Autodesk Inventor part; units mm, degrees
ref_plane "YZ Plane" through (0, 0, 0) normal (1, 0, 0) x (0, 1, 0)
ref_plane "XZ Plane" through (0, 0, 0) normal (0, 1, 0) x (-1, 0, 0)
ref_plane "XY Plane" through (0, 0, 0) normal (0, 0, 1) x (1, 0, 0)
sketch "Sketch1" plane through (0, 0, 0) normal (0, 0, 1) x (1, 0, 0)
  line L0 (0, 0) -> (20, 0)
  line L1 (20, 0) -> (20, 20)
  line L2 (20, 20) -> (0, 20)
  line L3 (0, 20) -> (0, 0)
  dimension "d0" = 20
  dimension "d1" = 20
extrude "Extrusion1" add sketch "Sketch1" along normal blind 20
sketch "Sketch2" plane through (0, 20, 0) normal (0, 1, 0) x (1, 0, 0)
  line L0 (20, 0) -> (0, 0)
  line L1 (20, 0) -> (20, -20)
  circle A0 centre (10, -5.8) radius 6.2
  dimension "d4" = 12.4
  dimension "d5" = 10
  dimension "d6" = 5.8
extrude "Extrusion2" cut sketch "Sketch2" against normal blind 20
sketch "Sketch5" plane through (0, 0, 0) normal (0, 0, -1) x (-1, 0, 0)
  line L0 (-12.1909, 0) -> (-12.1909, 20)
  line L1 (-20, 20) -> (-12.1909, 20)
  line L2 (-12.1909, 0) -> (-20, 0)
  line L3 (-16.2, 20) -> (-16.2, 0)
  point P0 (0, 0)
extrude "Extrusion3" cut sketch "Sketch5" against normal blind 5.8
sketch "Sketch6" plane through (0, 0, 0) normal (0, 0, -1) x (-1, 0, 0)
  line L0 (-7.8091, 20) -> (-7.8091, 0)
  line L1 (0, 0) -> (-7.8091, 0)
  line L2 (-7.8091, 20) -> (0, 20)
  line L3 (-3.8, 20) -> (-3.8, 0)
extrude "Extrusion4" cut sketch "Sketch6" against normal blind 5.8
properties part number "SupportBlocks"
Input: part model. Units: mm. Frame: model coordinates. A direction names the side the tool comes from. Coordinates: 2 decimals unless noted, no trailing zeros. Write each loop counter-clockwise with the first axis right and the second up, starting at its lowest first coordinate (ties: lowest second). Pieces come first, ordered by that corner, then holes. Notation, with made-up numbers: (3.25, 84.5) - (25.25, 84.5) arc R18 cw to (25.25, 94.5) - close; hole circle Ø5 at (63.25, 76). An arc over 180 degrees is marked (long way). Put each result on its own line as item: value. Start each with the question number.
1) Mould query, pull axis X, two halves, no side actions, for faces 3 (the face through (0, 10, 10)), 4 (the face through (3.8, 10, 3)), 5 (the face through (18, 10, 0)). Classes: pulls with the +X half, pulls with the -X half, needs draft (parallel to the pull), parting line crosses it, or undercut.
2) Cut plane B-B (y = 14.5). Return the cut outline in (x, z).
3) Ray query, L1, parallel to X at y = 10.25, z = 1; L2, parallel to X at y = 8.5, z = 9.5; L3, parallel to Z at x = 9, y = 14.25. Return the intervals inside material, ascending.
4) Cut plane A-A (z = 3.75). Return the cut outline in (x, y).
5) Contact query for a flat-ended pin moving along its axis: pin 1 (4 mm diameter, centred on x = 14, z = 5.5, fed in from +Y). Output: stop coordinate, or through.
6) Cut plane D-D (z = 10.5). Return the cut outline in (x, y).
7) Reachability of faces 1 (the face through (20, 10, 10)), 2 (the face through (16.2, 10, 3)) from +Z, -Z, +X, -X, +Y, -Y: full face, straight path, thin tool, end or side. Return the list, or none.
8) Cut plane C-C (x = 10). Return the cut outline in (y, z).
Resolved:
1. face 3: pulls with the -X half
1. face 4: undercut
1. face 5: needs draft
2. outline: (0, 0) - (3.8, 0) - (3.8, 5.8) arc R6.2 cw to (16.2, 5.8) - (16.2, 0) - (20, 0) - (20, 20) - (0, 20) - close
3. L1: x = 0 to 3.8, 16.2 to 20
3. L2: x = 0 to 5.03, 14.97 to 20
3. L3: z = 11.92 to 20
4. outline: (0, 0) - (3.8, 0) - (3.8, 20) - (0, 20) - close; (16.2, 0) - (20, 0) - (20, 20) - (16.2, 20) - close
5. pin 1: passes through
6. outline: (0, 0) - (5.96, 0) - (5.96, 20) - (0, 20) - close; (14.04, 0) - (20, 0) - (20, 20) - (14.04, 20) - close
7. face 1: +Z, -Z, +X, +Y, -Y
7. face 2: -Z, +Y, -Y
8. outline: (0, 12) - (20, 12) - (20, 20) - (0, 20) - close
